The drawing under review shows one solid part. Ordinate dimensions are in mm from its lowest x, y, z. A direction names the side the tool comes from. Coordinates: 2 decimals unless noted, no trailing zeros. Write each loop counter-clockwise with the first axis right and the second up, starting at its lowest first coordinate (ties: lowest second). Pieces come first, ordered by that corner, then holes.
1) Add section A-A, the plane z = 26. State the section outline as (x, y) points, then the cut area to 3 significant figures.
2) For P1, Ø10, axis at y = 20.5, z = 11.5, coming from the +X side; P2, Ø1.5, axis at x = 35.5, y = 30.5, coming from the -Z side (3 decimals); P3, Ø2, axis at y = 7.5, z = 10, coming from the -X side, all flat-tipped, find the tip position at first contact; note any pin that passes through.
3) Add section B-B, the plane y = 11. State the section outline as (x, z) points, then the cut area to 3 significant figures.
4) Add section C-C, the plane x = 11. State the section outline as (y, z) points.
5) Machinability: for the marked faces 1, 2 and 3, which of the approach directions +Z, -Z, +X, -X, +Y, -Y give a long, thin tool a straight path to every point of the face, cutting with its end or side? Answer none if there is none.
6) For line 1 (X direction, y = 34.5, z = 30); line 2 (Y direction, x = 32, z = 14); line 3 (Z direction, x = 25, y = 13), list the stretches that pass through material, from the lowest coordinate up.
7) Add section D-D, the plane z = 21. State the section outline as (x, y) points.
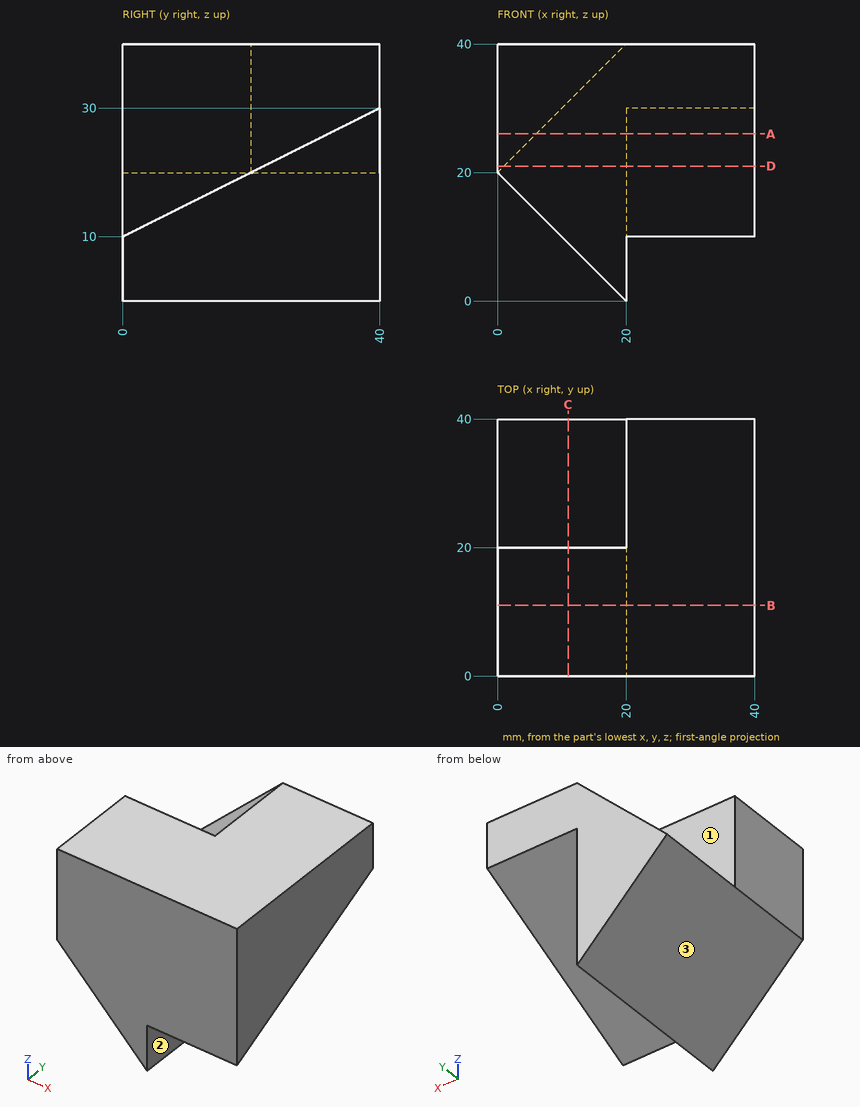
Geometry results:
1. outline: (0, 0) - (40, 0) - (40, 32) - (20, 32) - (20, 40) - (6, 40) - (6, 20) - (0, 20) - close
1. area: 1,320 mm2
2. P1: stops at x = 20
2. P2: stops at z = 24.875
2. P3: stops at x = 9
3. outline: (0, 20) - (20, 0) - (20, 15.5) - (40, 15.5) - (40, 40) - (0, 40) - close
3. area: 1,090 mm2
4. outline: (0, 9) - (40, 9) - (40, 31) - (20, 31) - (20, 40) - (0, 40) - close
5. face 1: +Z, -X, +Y
5. face 2: -Z, +X, +Y
5. face 3: -Z, -X, +Y, -Y
6. line 1: x = 10 to 40
6. line 2: y = 0 to 8
6. line 3: z = 16.5 to 40
7. outline: (0, 0) - (40, 0) - (40, 22) - (20, 22) - (20, 40) - (1, 40) - (1, 20) - (0, 20) - close
